The model under review builds one solid part; all positions refer to its coordinate system, in mm. A direction names the side the tool comes from. Round coordinates to 2 decimals unless told otherwise and drop trailing zeros. Write each loop counter-clockwise with the first axis right and the second up, starting at its lowest first coordinate (ties: lowest second). Pieces come first, ordered by that corner, then holes. Notation, with made-up numbers: (86, -32) -> (139, -32) arc R11 cw to (139, -15) -> close; hole circle Ø10 at (-38.75, 15.5). An arc over 180 degrees is marked (long way). Use CSV: the item, a comma, the result in double quotes. Start each with the question number.
1) Machinability: for faces 4 (the face through (-9.131, -17, 0)), 5 (the face through (0, -56.324, -5)), 6 (the face through (0, -56.324, 5)), 7 (the face through (-14.834, -34, 0)), which of the approach directions +Z, -Z, +X, -X, +Y, -Y give a long, thin tool a straight path to every point of the face, cutting with its end or side? Answer none if there is none.
2) Take a section at D-D, the plane x = 10.5. Give the boundary of the cut face in (y, z).
3) Take a section at B-B, the plane x = 0. Give the boundary of the cut face in (y, z).
4) Wall thickness on probe 1 along X at (y, z) = (-25, -1); probe 2 along Z at (x, y) = (0, -1.5); probe 3 along Y at (x, z) = (-6.25, 3.5): over which ranges is each line inside the solid? List them lowest first. Write a range as [from, to].
5) Take a section at A-A, the plane y = -9. Give the boundary of the cut face in (x, z), then the cut area to 3 significant figures.
6) For pin 1 Ø4 at (x, y) = (-5, -43.5) entering from -Z; pin 2 Ø15 at (x, y) = (5.5, -35.5) entering from +Z; pin 3 Ø1.5 at (y, z) = (-84.5, -7) entering from +X; pin 4 Ø1.5 at (y, z) = (-47.5, 3.5) entering from -X, all flat-tipped, find the tip position at first contact; note any pin that passes through.
7) Take a section at C-C, the plane x = -5. Give the boundary of the cut face in (y, z), then the cut area to 3 significant figures.
8) Mouldability with a two-part tool opening along X and no side actions: class faces 1 (the face through (-3, 0, 3)), 2 (the face through (-0.86, -3.394, -3.874)), 3 (the face through (-0.2, -3.4, -12.7)) as released by +X, released by -X, zero draft, split by the parting line, or undercut.
from build123d import *

# Parameters (mm, degrees)
F0_R          = 12.7
F0_R_2        = 3.96875
F1_DEPTH      = 6.8834
F3_DEPTH      = 2.6543
F4_T1_DEPTH   = 18.3727495789
F6_DEPTH      = 38.6842
F6_DEPTH_BACK = 10.16


# Not quite as in the source:
# - a fillet or chamfer that OpenCascade refuses, or shapes differently, is made with other operations: its cross-section is extruded or revolved along the edge and cut away or added


with BuildPart() as f1:
    # F0 (on Front) → F1 (new body)
    with BuildSketch(Plane.XZ):
        Circle(F0_R)
        Circle(F0_R_2, mode=Mode.SUBTRACT)
    extrude(amount=F1_DEPTH)

    # F2 (on Top) → F3 (join, symmetric)
    with BuildSketch(Plane.XY):
        Polygon((-9.1313, 0), (-14.8336, 0), (-14.8336, -66.4845), (14.8336, -66.4845), (14.8336, 0), (9.1313, 0), (9.1313, -26.3398), (-9.1313, -26.3398), align=None)
    extrude(amount=F3_DEPTH, both=True)

    # F4: chamfer of 2.54 on 2 edges, made by hand

    # F4_s2 → F4_t1 (cut)
    with BuildSketch(Plane.XY.offset(-9.1863747894)):
        Polygon((12.2936, 0), (14.8336, -2.54), (14.8336, 0), align=None)
        Polygon((-12.2936, 0), (-14.8336, -2.54), (-14.8336, 0), align=None)
    extrude(amount=F4_T1_DEPTH, mode=Mode.SUBTRACT)

    # F5 (on face) → F6 (join, two sides)
    with BuildSketch(Plane.XZ.offset(66.4845)) as f6_sk:
        with BuildLine():
            ThreePointArc((-7.4805479585, -2.6543), (0, -7.9375), (7.4805479585, -2.6543))
            Line((7.4805479585, -2.6543), (-7.4805479585, -2.6543))
        make_face()
        with BuildLine():
            ThreePointArc((7.4805479585, -2.6543), (7.8224278735, -1.3466730912), (7.9375, 0))
            ThreePointArc((7.9375, 0), (7.8224278735, 1.3466730912), (7.4805479585, 2.6543))
            Line((7.4805479585, 2.6543), (-7.4805479585, 2.6543))
            ThreePointArc((-7.4805479585, 2.6543), (-7.9375, 0), (-7.4805479585, -2.6543))
            Line((-7.4805479585, -2.6543), (7.4805479585, -2.6543))
        make_face()
        with BuildLine():
            Line((-7.4805479585, 2.6543), (7.4805479585, 2.6543))
            ThreePointArc((7.4805479585, 2.6543), (0, 7.9375), (-7.4805479585, 2.6543))
        make_face()
    extrude(amount=F6_DEPTH)
    extrude(f6_sk.sketch, amount=-F6_DEPTH_BACK)


solid = f1.part
Values found:
1,face 4,"+Z, -Z"
1,face 5,"-Z, +X, -X"
1,face 6,"+Z, +X, -X"
1,face 7,"+Z, -Z, -X, +Y, -Y"
2,outline,"(-66.48, -2.65) -> (-6.88, -2.65) -> (-6.88, -7.14) -> (0, -7.14) -> (0, 7.14) -> (-6.88, 7.14) -> (-6.88, 2.65) -> (-66.48, 2.65) -> close"
3,outline,"(-105.17, -7.94) -> (-56.32, -7.94) -> (-56.32, -2.65) -> (-26.34, -2.65) -> (-26.34, 2.65) -> (-56.32, 2.65) -> (-56.32, 7.94) -> (-105.17, 7.94) -> close; (-6.88, -12.7) -> (0, -12.7) -> (0, -3.97) -> (-6.88, -3.97) -> close; (-6.88, 3.97) -> (0, 3.97) -> (0, 12.7) -> (-6.88, 12.7) -> close"
4,probe 1,"[-14.83, -9.13], [9.13, 14.83]"
4,probe 2,"[-12.7, -3.97], [3.97, 12.7]"
4,probe 3,"[-105.17, -56.32], [-6.88, 0]"
5,outline,"(-14.83, -2.65) -> (-9.13, -2.65) -> (-9.13, 2.65) -> (-14.83, 2.65) -> close; (9.13, -2.65) -> (14.83, -2.65) -> (14.83, 2.65) -> (9.13, 2.65) -> close"
5,area,"60.5 mm²"
6,pin 1,"z = -2.65"
6,pin 2,"z = 2.65"
6,pin 3,"x = 4.89"
6,pin 4,"through"
7,outline,"(-105.17, -6.16) -> (-56.32, -6.16) -> (-56.32, -2.65) -> (-26.34, -2.65) -> (-26.34, 2.65) -> (-56.32, 2.65) -> (-56.32, 6.16) -> (-105.17, 6.16) -> close; (-6.88, -11.67) -> (0, -11.67) -> (0, 11.67) -> (-6.88, 11.67) -> close"
7,area,"922 mm²"
8,face 1,"zero draft"
8,face 2,"undercut"
8,face 3,"split by the parting line"
